Model file for the job. Use its own axes, mm. Face numbers are marked on the shaded views. A direction names the side the tool comes from. Coordinates: 2 decimals unless noted, no trailing zeros. Write each loop counter-clockwise with the first axis right and the second up, starting at its lowest first coordinate (ties: lowest second). Pieces come first, ordered by that corner, then holes. Notation, with made-up numbers: (78.25, -35.5) -> (107.25, -35.5) arc R24 ccw to (107.25, -9.5) -> close; hole circle Ø11 at (63.25, 9). An arc over 180 degrees is marked (long way). Write item = value, one per line. Start each with the question number.
from build123d import *

# Parameters (mm, degrees)
SKETCH1_R           = 1.65
SKETCH1_W           = 19
SKETCH1_H           = 46
BOSS_EXTRUDE3_DEPTH = 5
CHAMFER1_SIZE       = 10
SKETCH6_W           = 10
SKETCH6_H           = 15
BOSS_EXTRUDE4_DEPTH = 20
SKETCH8_W           = 16
SKETCH8_H           = 21
SKETCH8_W_2         = 10
SKETCH8_H_2         = 15
BOSS_EXTRUDE5_DEPTH = 15
SKETCH5_W           = 16
SKETCH5_H           = 10.2
CUT_EXTRUDE1_DEPTH  = 64.492125496


with BuildPart() as part:
    # Sketch1 → Boss-Extrude3 (new body)
    with BuildSketch(Plane(origin=(0, 0, 0), x_dir=(1, 0, 0), z_dir=(0, 1, 0))):
        Polygon((42.5, 40), (-42.5, 40), (-42.5, 24.25), (-42.5, -24.25), (-42.5, -40), (-20, -40), (20, -40), (42.5, -40), (42.5, -24.25), (42.5, 24.25), align=None)
        with Locations(Location((-29.5, -32, 0), (0, 0, 270))):
            Circle(SKETCH1_R, mode=Mode.SUBTRACT)
        with Locations(Location((-19.5, -32, 0), (0, 0, 270))):
            Circle(SKETCH1_R, mode=Mode.SUBTRACT)
        with Locations(Location((19.5, -32, 0), (0, 0, 270))):
            Circle(SKETCH1_R, mode=Mode.SUBTRACT)
        with Locations(Location((29.5, -32, 0), (0, 0, 270))):
            Circle(SKETCH1_R, mode=Mode.SUBTRACT)
        Rectangle(SKETCH1_W, SKETCH1_H, mode=Mode.SUBTRACT)
        with Locations(Location((-29.5, 32, 0), (0, 0, 270))):
            Circle(SKETCH1_R, mode=Mode.SUBTRACT)
        with Locations(Location((-19.5, 32, 0), (0, 0, 270))):
            Circle(SKETCH1_R, mode=Mode.SUBTRACT)
        with Locations(Location((19.5, 32, 0), (0, 0, 270))):
            Circle(SKETCH1_R, mode=Mode.SUBTRACT)
        with Locations(Location((29.5, 32, 0), (0, 0, 270))):
            Circle(SKETCH1_R, mode=Mode.SUBTRACT)
    extrude(amount=BOSS_EXTRUDE3_DEPTH)

    # Chamfer1
    chamfer1_edges = [part.edges().sort_by_distance(p)[0] for p in [
        (-42.5, 2.5, 40),
        (42.5, 2.5, 40),
    ]]
    chamfer(chamfer1_edges, length=CHAMFER1_SIZE)

    # Sketch6 → Boss-Extrude4 (add)
    with BuildSketch(Plane(origin=(0, 5, 0), x_dir=(1, 0, 0), z_dir=(0, 1, 0))):
        with Locations((19.6, 15.6)):
            Rectangle(SKETCH6_W, SKETCH6_H)
        with Locations((-19.6, 15.6)):
            Rectangle(SKETCH6_W, SKETCH6_H)
        with Locations((-19.6, -15.6)):
            Rectangle(SKETCH6_W, SKETCH6_H)
        with Locations((19.6, -15.6)):
            Rectangle(SKETCH6_W, SKETCH6_H)
    extrude(amount=BOSS_EXTRUDE4_DEPTH)

    # Sketch8 → Boss-Extrude5 (add)
    # profile 1 of 4: a face of its own
    with BuildSketch(Plane(origin=(0, 5, 0), x_dir=(1, 0, 0), z_dir=(0, 1, 0))):
        with Locations((-19.6, 15.6)):
            Rectangle(SKETCH8_W, SKETCH8_H)
        with Locations((-19.6, 15.6)):
            Rectangle(SKETCH8_W_2, SKETCH8_H_2, mode=Mode.SUBTRACT)
    # profile 2 of 4: a face of its own
    with BuildSketch(Plane(origin=(0, 5, 0), x_dir=(1, 0, 0), z_dir=(0, 1, 0))):
        with Locations((-19.6, -15.6)):
            Rectangle(SKETCH8_W, SKETCH8_H)
        with Locations((-19.6, -15.6)):
            Rectangle(SKETCH8_W_2, SKETCH8_H_2, mode=Mode.SUBTRACT)
    # profile 3 of 4: a face of its own
    with BuildSketch(Plane(origin=(0, 5, 0), x_dir=(1, 0, 0), z_dir=(0, 1, 0))):
        with Locations((19.6, -15.6)):
            Rectangle(SKETCH8_W, SKETCH8_H)
        with Locations((19.6, -15.6)):
            Rectangle(SKETCH8_W_2, SKETCH8_H_2, mode=Mode.SUBTRACT)
    # profile 4 of 4: a face of its own
    with BuildSketch(Plane(origin=(0, 5, 0), x_dir=(1, 0, 0), z_dir=(0, 1, 0))):
        with Locations((19.6, 15.6)):
            Rectangle(SKETCH8_W, SKETCH8_H)
        with Locations((19.6, 15.6)):
            Rectangle(SKETCH8_W_2, SKETCH8_H_2, mode=Mode.SUBTRACT)
    extrude(amount=BOSS_EXTRUDE5_DEPTH)

    # Sketch5 → Cut-Extrude1 (cut, through all)
    with BuildSketch(Plane.XZ):
        with Locations((22.5, 0)):
            Rectangle(SKETCH5_W, SKETCH5_H)
    extrude(amount=-CUT_EXTRUDE1_DEPTH, mode=Mode.SUBTRACT)


solid = part.part
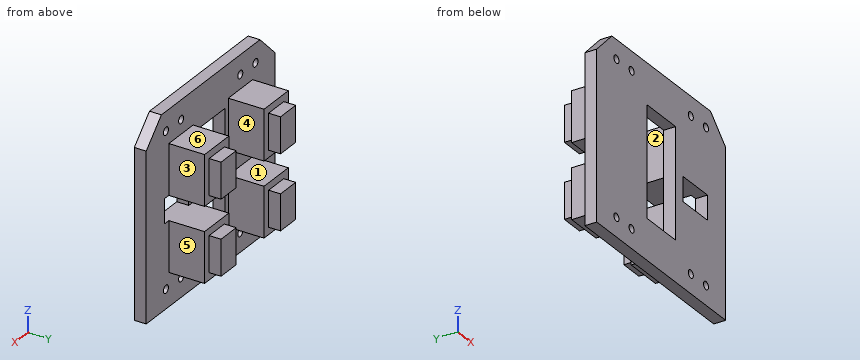
(1) 3-axis set-ups, long thin cutter, end or side, ignore diameter. For the marked faces 1, 2 and 3: which of +Z, -Z, +X, -X, +Y, -Y reach the whole face in a straight line?
(2) Saw through at A-A (z = -32). Give the cut face in (x, y).
(3) Drop flat-ended pins along their axis: pin 1 Ø5 at (y, z) = (22, 11.5) entering from +X; pin 2 Ø3 at (x, z) = (9.5, -19) entering from -Y; pin 3 Ø4.5 at (x, z) = (-29.5, -32) entering from +Y; pin 4 Ø7.5 at (y, z) = (10, -13.5) entering from -X. Give the stop position or say it passes through.
(4) Drill centre lines: line 1 along X through (y, z) = (1.55, -32); line 2 along X through (y, z) = (1.5, 3); line 3 along X through (y, z) = (17.75, -5.5). Where is each one in solid material? Low to high.
(5) Saw through at B-B (y = 10.5). Give the cut face in (x, z).
(6) Saw through at D-D (z = 18.5). Give the cut face in (x, y).
(7) Mould opens along X. For the marked faces 4, 5 and 6 say: released by +X, released by -X, zero draft, split by the parting line, or undercut.
(8) Saw through at C-C (x = -29.5). Give the cut face in (y, z), then the cut area to 3 significant figures.
Returned:
q1.face_1 = +X, -X, +Y
q1.face_2 = +Z, -Z, +Y
q1.face_3 = +Z, -Z, +X, +Y
q2.outline = (-42.5, 0) -> (-31.15, 0) -> (-31.15, 5) -> (-42.5, 5) -> close; (-27.85, 0) -> (-21.15, 0) -> (-21.15, 5) -> (-27.85, 5) -> close; (-17.85, 0) -> (17.85, 0) -> (17.85, 5) -> (-17.85, 5) -> close; (21.15, 0) -> (27.85, 0) -> (27.85, 5) -> (21.15, 5) -> close; (31.15, 0) -> (42.5, 0) -> (42.5, 5) -> (31.15, 5) -> close
q3.pin_1 = 27.6
q3.pin_2 = 0
q3.pin_3 = 5
q3.pin_4 = -27.6
q4.line_1 = -42.5 to -31.15, -27.85 to -21.15, -17.85 to 17.85, 21.15 to 27.85, 31.15 to 42.5
q4.line_2 = -42.5 to -9.5, 9.5 to 14.5, 30.5 to 42.5
q4.line_3 = -27.6 to -11.6, 11.6 to 27.6
q5.outline = (-27.6, -26.1) -> (-11.6, -26.1) -> (-11.6, -5.1) -> (-27.6, -5.1) -> close; (-27.6, 5.1) -> (-11.6, 5.1) -> (-11.6, 26.1) -> (-27.6, 26.1) -> close; (11.6, -26.1) -> (27.6, -26.1) -> (27.6, -5.1) -> (11.6, -5.1) -> close; (11.6, 5.1) -> (27.6, 5.1) -> (27.6, 26.1) -> (11.6, 26.1) -> close
q6.outline = (-42.5, 0) -> (-9.5, 0) -> (-9.5, 5) -> (-11.6, 5) -> (-11.6, 20) -> (-14.6, 20) -> (-14.6, 25) -> (-24.6, 25) -> (-24.6, 20) -> (-27.6, 20) -> (-27.6, 5) -> (-42.5, 5) -> close; (9.5, 0) -> (42.5, 0) -> (42.5, 5) -> (27.6, 5) -> (27.6, 20) -> (24.6, 20) -> (24.6, 25) -> (14.6, 25) -> (14.6, 20) -> (11.6, 20) -> (11.6, 5) -> (9.5, 5) -> close
q7.face_4 = undercut
q7.face_5 = released by +X
q7.face_6 = zero draft
q8.outline = (0, -40) -> (5, -40) -> (5, -33.65) -> (0, -33.65) -> close; (0, -30.35) -> (5, -30.35) -> (5, 30.35) -> (0, 30.35) -> close; (0, 33.65) -> (5, 33.65) -> (5, 40) -> (0, 40) -> close
q8.area = 367 mm2
